The figure shows three views and two pictorial views of one solid part (mm, origin at its lowest corner). Answer the questions. Coordinates: 2 decimals unless noted, no trailing zeros. Order: outer loops, then holes, each group sorted by start corner. A loop starts at its lowest first (then second) coordinate and runs counter-clockwise, first axis right, second up. Notation, with made-up numbers: (-24, -3.75) - (-1, -3.75) arc R17 cw to (-1, 23.25) - close; hole circle Ø3 at (-18.75, 44). An arc over 180 degrees is marked (long way). Use one line per item in the form item = value. Start each with the question number.
Item 1: Each of these flat-tipped pins is pushed along its axis until it touches: pin 1 Ø6.5 at (x, y) = (9, 15.65) entering from +Z; pin 2 Ø9 at (x, y) = (10.5, 14.5) entering from +Z. Where does it stop, or does it pass through?
Item 2: Section C-C, the plane y = 15.65 is taken. Write down the section's boundary in (x, z), and give its area (3 significant figures).
Item 3: Consider line 1 along Y through (x, z) = (4, 27); line 2 along Y through (x, z) = (1.5, 50); line 3 along X through (y, z) = (26, 66.5). Determine where each line is inside the solid, lowest interval first. Write a range as [from, to].
Item 4: Section D-D, the plane y = 6 is taken. Write down the section's boundary in (x, z).
Item 5: Section B-B, the plane x = 9 is taken. Write down the section's boundary in (y, z).
Item 6: Section A-A, the plane z = 51 is taken. Write down the section's boundary in (x, y).
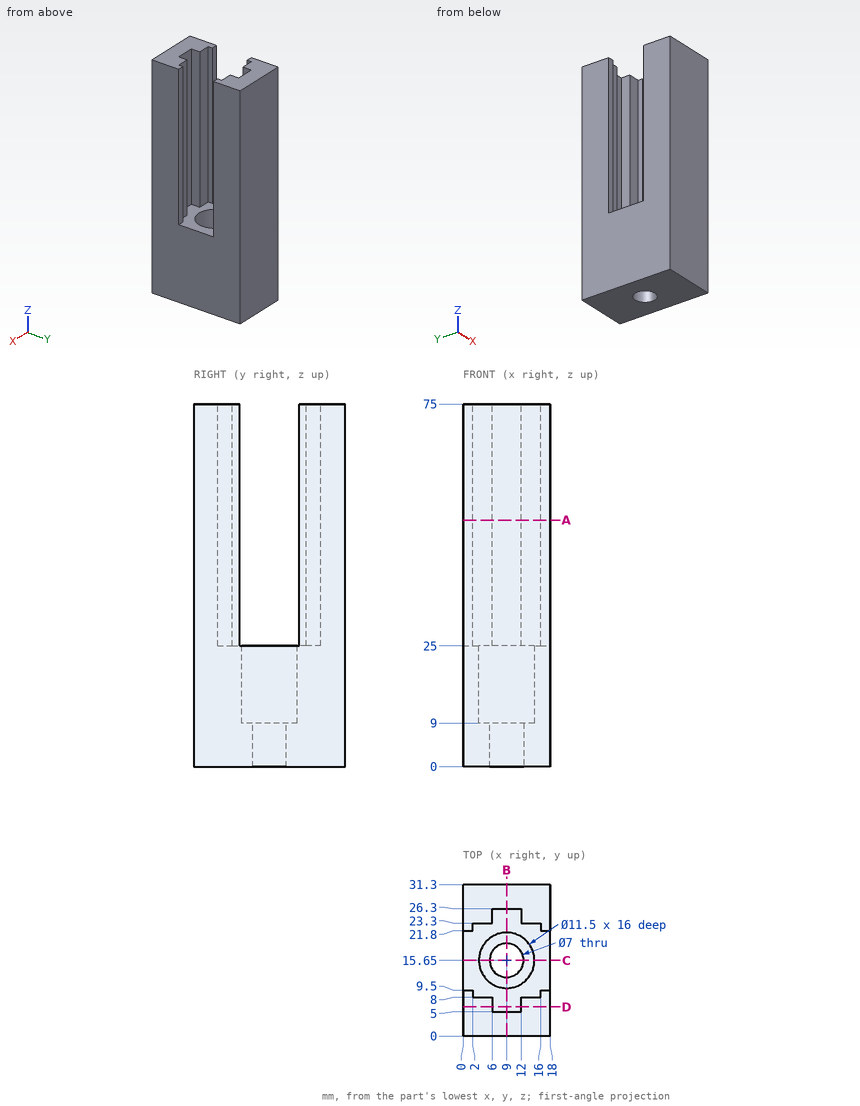
Response:
q1.pin_1 = through
q1.pin_2 = 25
q2.outline = (0, 0) - (5.5, 0) - (5.5, 9) - (3.25, 9) - (3.25, 25) - (0, 25) - close; (12.5, 0) - (18, 0) - (18, 25) - (14.75, 25) - (14.75, 9) - (12.5, 9) - close
q2.area = 203 mm2
q3.line_1 = [0, 8], [23.3, 31.3]
q3.line_2 = [0, 9.5], [21.8, 31.3]
q3.line_3 = [0, 6], [12, 18]
q4.outline = (0, 0) - (18, 0) - (18, 75) - (12, 75) - (12, 25) - (6, 25) - (6, 75) - (0, 75) - close
q5.outline = (0, 0) - (12.15, 0) - (12.15, 9) - (9.9, 9) - (9.9, 25) - (5, 25) - (5, 75) - (0, 75) - close; (19.15, 0) - (31.3, 0) - (31.3, 75) - (26.3, 75) - (26.3, 25) - (21.4, 25) - (21.4, 9) - (19.15, 9) - close
q6.outline = (0, 0) - (18, 0) - (18, 9.5) - (16, 9.5) - (16, 8) - (12, 8) - (12, 5) - (6, 5) - (6, 8) - (2, 8) - (2, 9.5) - (0, 9.5) - close; (0, 21.8) - (2, 21.8) - (2, 23.3) - (6, 23.3) - (6, 26.3) - (12, 26.3) - (12, 23.3) - (16, 23.3) - (16, 21.8) - (18, 21.8) - (18, 31.3) - (0, 31.3) - close
